Source: CAD feature listing. Evaluate the final solid. Frame: model axes, mm. A direction names the side the tool comes from. Give positions to 0.01 mm unless a question says otherwise; leave off trailing zeros. Write each loop counter-clockwise with the first axis right and the second up, starting at its lowest first coordinate (ties: lowest second). Pieces come first, ordered by that corner, then holes.
```python
from build123d import *

# Parameters (mm, degrees)
F0_W     = 3.81
F0_H     = 19.05
F1_DEPTH = 3.429


# Not quite as in the source:
# - ends of sketch curves that miss each other by under 0.0002 mm in the source are joined


with BuildPart() as f1:
    # F0 (on Front) → F1 (new body)
    with BuildSketch(Plane.XZ):
        Polygon((65.6458174, -303.6329462), (62.4708174, -303.6329462), (62.4708174, -321.4129462), (65.6458174, -321.4129462), (65.6458174, -356.9729462), (124.8784904, -393.99337), (123.1957404, -396.68577), (138.273155, -406.1091446), (139.955905, -403.4167446), (194.5357298, -437.5291224), (192.8529798, -440.2215224), (207.9303944, -449.644897), (209.6131444, -446.9525224), (268.8458174, -483.9729462), (339.9658174, -483.9729462), (339.9658174, -487.1479462), (357.7458174, -487.1479462), (357.7458174, -483.9729462), (560.9458174, -483.9729462), (560.9458174, -487.1479462), (578.7258174, -487.1479462), (578.7258174, -483.9729462), (649.8458174, -483.9729462), (709.0784904, -446.9525224), (710.7612404, -449.644897), (725.838655, -440.2215224), (724.155905, -437.5291224), (778.7357298, -403.4167446), (780.4184798, -406.1091446), (795.495869, -396.68577), (793.8131444, -393.99337), (853.0458174, -356.9729462), (853.0458174, -321.4129462), (856.2208174, -321.4129462), (856.2208174, -303.6329462), (853.0458174, -303.6329462), (853.0458174, -268.0729462), (776.8458174, -268.0729462), (776.8458174, -264.8979462), (759.0658174, -264.8979462), (759.0658174, -268.0729462), (549.5158174, -268.0729462), (549.5158174, -433.1729462), (514.5908174, -433.1729462), (514.5908174, -268.0729462), (468.2358174, -268.0729462), (468.2358174, -264.8979462), (450.4558174, -264.8979462), (450.4558174, -268.0729462), (159.6258174, -268.0729462), (159.6258174, -264.8979462), (141.8458174, -264.8979462), (141.8458174, -268.0729462), (65.6458174, -268.0729462), align=None)
        with Locations((346.6968174, -443.3329462)):
            Rectangle(F0_W, F0_H, mode=Mode.SUBTRACT)
        with BuildLine():
            ThreePointArc((372.0333174, -442.6979462), (376.7958174, -437.9354462), (381.5583174, -442.6979462))
            Line((381.5583174, -442.6979462), (381.5583174, -474.4479462))
            ThreePointArc((381.5583174, -474.4479462), (376.7958174, -479.2104462), (372.0333174, -474.4479462))
            Line((372.0333174, -474.4479462), (372.0333174, -442.6979462))
        make_face(mode=Mode.SUBTRACT)
        with BuildLine():
            ThreePointArc((457.7583174, -474.4479462), (452.9958174, -479.2104462), (448.2333174, -474.4479462))
            Line((448.2333174, -474.4479462), (448.2333174, -442.6979462))
            ThreePointArc((448.2333174, -442.6979462), (452.9958174, -437.9354462), (457.7583174, -442.6979462))
            Line((457.7583174, -442.6979462), (457.7583174, -474.4479462))
        make_face(mode=Mode.SUBTRACT)
        with Locations((197.3448174, -397.6129462)):
            Rectangle(F0_W, F0_H, mode=Mode.SUBTRACT)
        with Locations((571.9948174, -443.3329462)):
            Rectangle(F0_W, F0_H, mode=Mode.SUBTRACT)
        with Locations((721.3468174, -397.6129462)):
            Rectangle(F0_W, F0_H, mode=Mode.SUBTRACT)
        with BuildLine():
            ThreePointArc((179.9458174, -356.5983978), (170.1306614744, -373.26033511), (150.7993444424, -372.7527697722))
            Line((150.7993444424, -372.7527697722), (106.3493428, -344.9715224))
            ThreePointArc((106.3493428, -344.9715224), (99.78388009, -338.0519918744), (97.3958174, -328.8171478))
            Line((97.3958174, -328.8171478), (97.3958174, -318.8729462))
            ThreePointArc((97.3958174, -318.8729462), (102.9754332184, -305.4025620184), (116.4458174, -299.8229462))
            Line((116.4458174, -299.8229462), (160.8958174, -299.8229462))
            ThreePointArc((160.8958174, -299.8229462), (174.3662015816, -305.4025620184), (179.9458174, -318.8729462))
            Line((179.9458174, -318.8729462), (179.9458174, -356.5983978))
        make_face(mode=Mode.SUBTRACT)
        with BuildLine():
            ThreePointArc((226.9993444424, -420.3777697722), (220.43388009, -413.4582418744), (218.0458174, -404.2233978))
            Line((218.0458174, -404.2233978), (218.0458174, -318.8729462))
            ThreePointArc((218.0458174, -318.8729462), (223.6254332184, -305.4025620184), (237.0958174, -299.8229462))
            Line((237.0958174, -299.8229462), (294.2458174, -299.8229462))
            ThreePointArc((294.2458174, -299.8229462), (307.7162015816, -305.4025620184), (313.2958174, -318.8729462))
            Line((313.2958174, -318.8729462), (313.2958174, -433.1729462))
            ThreePointArc((313.2958174, -433.1729462), (307.7162015816, -446.6433303816), (294.2458174, -452.2229462))
            Line((294.2458174, -452.2229462), (283.4150542, -452.2229462))
            ThreePointArc((283.4150542, -452.2229462), (278.1632997385, -451.4847340722), (273.3185698266, -449.3273110374))
            Line((273.3185698266, -449.3273110374), (226.9993444424, -420.3777697722))
        make_face(mode=Mode.SUBTRACT)
        with Locations((197.3448174, -308.7129462)):
            Rectangle(F0_W, F0_H, mode=Mode.SUBTRACT)
        with Locations((346.6968174, -308.7129462)):
            Rectangle(F0_W, F0_H, mode=Mode.SUBTRACT)
        with BuildLine():
            ThreePointArc((372.0333174, -280.7729462), (376.7958174, -276.0104462), (381.5583174, -280.7729462))
            Line((381.5583174, -280.7729462), (381.5583174, -312.5229462))
            ThreePointArc((381.5583174, -312.5229462), (376.7958174, -317.2854462), (372.0333174, -312.5229462))
            Line((372.0333174, -312.5229462), (372.0333174, -280.7729462))
        make_face(mode=Mode.SUBTRACT)
        with BuildLine():
            ThreePointArc((457.7583174, -312.5229462), (452.9958174, -317.2854462), (448.2333174, -312.5229462))
            Line((448.2333174, -312.5229462), (448.2333174, -280.7729462))
            ThreePointArc((448.2333174, -280.7729462), (452.9958174, -276.0104462), (457.7583174, -280.7729462))
            Line((457.7583174, -280.7729462), (457.7583174, -312.5229462))
        make_face(mode=Mode.SUBTRACT)
        with BuildLine():
            ThreePointArc((624.4458174, -452.2229462), (610.9754332184, -446.6433303816), (605.3958174, -433.1729462))
            Line((605.3958174, -433.1729462), (605.3958174, -318.8729462))
            ThreePointArc((605.3958174, -318.8729462), (610.9754332184, -305.4025620184), (624.4458174, -299.8229462))
            Line((624.4458174, -299.8229462), (681.5958174, -299.8229462))
            ThreePointArc((681.5958174, -299.8229462), (695.0662015816, -305.4025620184), (700.6458174, -318.8729462))
            Line((700.6458174, -318.8729462), (700.6458174, -404.2233978))
            ThreePointArc((700.6458174, -404.2233978), (698.25775471, -413.4582418744), (691.6922903576, -420.3777697722))
            Line((691.6922903576, -420.3777697722), (645.3730552, -449.3272954))
            ThreePointArc((645.3730552, -449.3272954), (640.5283200138, -451.4847311032), (635.2765552, -452.2229462))
            Line((635.2765552, -452.2229462), (624.4458174, -452.2229462))
        make_face(mode=Mode.SUBTRACT)
        with BuildLine():
            ThreePointArc((738.7458174, -318.8729462), (744.3254332184, -305.4025620184), (757.7958174, -299.8229462))
            Line((757.7958174, -299.8229462), (802.2458174, -299.8229462))
            ThreePointArc((802.2458174, -299.8229462), (815.7162015816, -305.4025620184), (821.2958174, -318.8729462))
            Line((821.2958174, -318.8729462), (821.2958174, -328.8171478))
            ThreePointArc((821.2958174, -328.8171478), (818.90775471, -338.0519918744), (812.3422903576, -344.9715197722))
            Line((812.3422903576, -344.9715197722), (767.892292, -372.7527724))
            ThreePointArc((767.892292, -372.7527724), (748.5609733256, -373.26033511), (738.7458174, -356.5983978))
            Line((738.7458174, -356.5983978), (738.7458174, -318.8729462))
        make_face(mode=Mode.SUBTRACT)
        with Locations((571.9948174, -308.7129462)):
            Rectangle(F0_W, F0_H, mode=Mode.SUBTRACT)
        with Locations((721.3468174, -308.7129462)):
            Rectangle(F0_W, F0_H, mode=Mode.SUBTRACT)
    extrude(amount=F1_DEPTH)


solid = f1.part
```
1. Line query: L1, parallel to X at y = -2.4, z = -281; L2, parallel to X at y = -2.75, z = -324; L3, parallel to X at y = -0.4, z = -474. Output: solid intervals per line, ascending.
2. Contact query for flat-ended pins moving along their axis: P1, Ø1, axis at x = 360.5, y = -0.5, coming from the -Z side; P2, Ø1, axis at x = 492.5, y = -1.5, coming from the +Z side; P3, Ø1.5, axis at y = -2.5, z = -443, coming from the -X side. Output: stop coordinate, or through.
3. Access query for faces 1 (the flat face through (790.428, -1.69, -358.668)), 2 (the flat face through (454, 0, -350)). Directions: +Z, -Z, +X, -X, +Y, -Y. A direction counts if a zero-diameter tool reaches every point of the face in a straight line with its end or side. Return the directions, or none.
4. Mould query, pull axis X, two halves, no side actions, for faces 3 (the cylindrical face through (610.83, -1.69, -305.55)), 4 (the flat face through (454, -3.429, -350)), 5 (the cylindrical face through (307.57, -1.69, -305.26)), 6 (the flat face through (823.015, -1.69, -375.742)). Classes: +X half, -X half, draft (parallel to the pull), parting line (faces both ways), or undercut.
5. Cut plane A-A, the plane x = 251. Return the cut outline in (y, z).
6. Cut plane B-B, the plane y = -1.85. State how many separate pieces and enclosed holes the cut face has, then the cut area to 3 significant figures.
Response values:
1. L1: x = 65.65 to 372.03, 381.56 to 448.23, 457.76 to 514.59, 549.52 to 853.05
1. L2: x = 65.65 to 97.4, 179.95 to 218.05, 313.3 to 514.59, 549.52 to 605.4, 700.65 to 738.75, 821.3 to 853.05
1. L3: x = 252.89 to 372.03, 381.56 to 448.23, 457.76 to 665.8
2. P1: stops at z = -483.97
2. P2: stops at z = -268.07
2. P3: stops at x = 196.1
3. face 1: +Y, -Y
3. face 2: +Z, -Z, +X, -X, +Y
4. face 3: undercut
4. face 4: draft
4. face 5: undercut
4. face 6: +X half
5. outline: (-3.43, -472.82) - (0, -472.82) - (0, -435.38) - (-3.43, -435.38) - close; (-3.43, -299.82) - (0, -299.82) - (0, -268.07) - (-3.43, -268.07) - close
6. separate pieces: 1
6. enclosed holes: 16
6. area: 101,000 mm2
